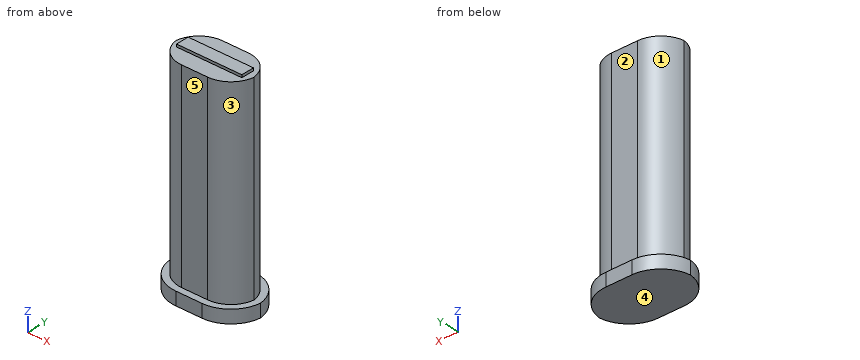
from build123d import *

# Parameters (mm, degrees)
F0_W     = 12.7
F0_H     = 2.54
F1_DEPTH = 38.608
F2_DEPTH = 38.1
F3_DEPTH = 2.54


with BuildPart() as f1:
    # F0 (on Top) → F1 (new body)
    with BuildSketch(Plane.XY):
        Rectangle(F0_W, F0_H)
    extrude(amount=F1_DEPTH)



with BuildPart() as f2:
    # F0 (on Top) → F2 (new body)
    with BuildSketch(Plane.XY):
        with BuildLine():
            Line((-2.54, -4.445), (2.54, -4.445))
            ThreePointArc((2.54, -4.445), (5.900104, -3.175), (7.580156, 0))
            ThreePointArc((7.580156, 0), (5.900104, 3.175), (2.54, 4.445))
            Line((2.54, 4.445), (-2.54, 4.445))
            ThreePointArc((-2.54, 4.445), (-5.900104, 3.175), (-7.580156, 0))
            ThreePointArc((-7.580156, 0), (-5.900104, -3.175), (-2.54, -4.445))
        make_face()
        Rectangle(F0_W, F0_H, mode=Mode.SUBTRACT)
        Rectangle(F0_W, F0_H)
    extrude(amount=F2_DEPTH)


with BuildPart() as f1_1:
    add(f1.part)

    add(f2.part)  # F3 merges F2
    # F0 (on Top) → F3 (join)
    with BuildSketch(Plane.XY):
        with BuildLine():
            Line((-2.54, -5.715), (2.54, -5.715))
            ThreePointArc((2.54, -5.715), (6.799709, -4.074286), (8.85817, 0))
            ThreePointArc((8.85817, 0), (6.799709, 4.074286), (2.54, 5.715))
            Line((2.54, 5.715), (-2.54, 5.715))
            ThreePointArc((-2.54, 5.715), (-6.799709, 4.074286), (-8.85817, 0))
            ThreePointArc((-8.85817, 0), (-6.799709, -4.074286), (-2.54, -5.715))
        make_face()
        with BuildLine():
            ThreePointArc((-7.62, 0.635), (-7.610029, 0.316876), (-7.580156, 0))
            ThreePointArc((-7.580156, 0), (-7.610029, -0.316876), (-7.62, -0.635))
            Line((-7.62, -0.635), (-7.62, 0.635))
        make_face(mode=Mode.SUBTRACT)
        with BuildLine():
            ThreePointArc((7.580156, 0), (5.900104, -3.175), (2.54, -4.445))
            Line((2.54, -4.445), (-2.54, -4.445))
            ThreePointArc((-2.54, -4.445), (-5.900104, -3.175), (-7.580156, 0))
            ThreePointArc((-7.580156, 0), (-5.900104, 3.175), (-2.54, 4.445))
            Line((-2.54, 4.445), (2.54, 4.445))
            ThreePointArc((2.54, 4.445), (5.900104, 3.175), (7.580156, 0))
        make_face(mode=Mode.SUBTRACT)
        with BuildLine():
            ThreePointArc((7.62, -0.635), (7.610029, -0.316876), (7.580156, 0))
            ThreePointArc((7.580156, 0), (7.610029, 0.316876), (7.62, 0.635))
            Line((7.62, 0.635), (7.62, -0.635))
        make_face(mode=Mode.SUBTRACT)
        with BuildLine():
            Line((-2.54, -4.445), (2.54, -4.445))
            ThreePointArc((2.54, -4.445), (5.900104, -3.175), (7.580156, 0))
            ThreePointArc((7.580156, 0), (5.900104, 3.175), (2.54, 4.445))
            Line((2.54, 4.445), (-2.54, 4.445))
            ThreePointArc((-2.54, 4.445), (-5.900104, 3.175), (-7.580156, 0))
            ThreePointArc((-7.580156, 0), (-5.900104, -3.175), (-2.54, -4.445))
        make_face()
        Rectangle(F0_W, F0_H, mode=Mode.SUBTRACT)
        Rectangle(F0_W, F0_H)
        with BuildLine():
            ThreePointArc((7.62, 0.635), (7.610029, 0.316876), (7.580156, 0))
            ThreePointArc((7.580156, 0), (7.610029, -0.316876), (7.62, -0.635))
            Line((7.62, -0.635), (7.62, 0.635))
        make_face()
        with BuildLine():
            ThreePointArc((-7.62, -0.635), (-7.610029, -0.316876), (-7.580156, 0))
            ThreePointArc((-7.580156, 0), (-7.610029, 0.316876), (-7.62, 0.635))
            Line((-7.62, 0.635), (-7.62, -0.635))
        make_face()
    extrude(amount=-F3_DEPTH)


solid = f1_1.part
The listing builds one solid part. Answer for the finished solid, in the listing's coordinates (mm). Face numbers are marked on the shaded views. A direction names the side the tool comes from. Give positions to 0.01 mm unless a question says otherwise; leave off trailing zeros. Loops run counter-clockwise (first coordinate to the right, second up) from the corner with the lowest first, then second, coordinate; pieces in that order, holes last. Notation, with made-up numbers: (-18.5, 48.5) - (-2.5, 48.5) arc R19 ccw to (-2.5, 75.5) - close; hole circle Ø11 at (-7.5, 46.25). An arc over 180 degrees is marked (long way). Answer as a JSON object with one key per item and string values.
1. A cutting plane is placed at D-D (x = -3.5). Write down the section's boundary in (y, z).
Determined:
{"outline": "(-5.64, -2.54) - (5.64, -2.54) - (5.64, 0) - (4.35, 0) - (4.35, 38.1) - (1.27, 38.1) - (1.27, 38.61) - (-1.27, 38.61) - (-1.27, 38.1) - (-4.35, 38.1) - (-4.35, 0) - (-5.64, 0) - close"}
2. For the marked faces 1, 2, 3, 4 and 5, determine the directions among +Z, -Z, +X, -X, +Y, -Y from which every point of the face is accessible in a straight line to the end or side of a thin tool.
Determined:
{"face 1": "+Z, -X, +Y", "face 2": "+Z, +X, -X, +Y", "face 3": "+Z, +X, -Y", "face 4": "-Z, +X, -X, +Y, -Y", "face 5": "+Z, +X, -X, -Y"}
3. Flat-ended cylindrical pins translate along their axes: pin 1 Ø1 at (y, z) = (4.5, 31) entering from +X; pin 2 Ø5 at (x, z) = (-1.5, 12.5) entering from -Y (3 decimals); pin 3 Ø0.6 at (x, z) = (1, 38.5) entering from -Y. Find the tip coordinate at first contact, or state that the pin passes through.
Determined:
{"pin 1": "x = 4.62", "pin 2": "y = -4.445", "pin 3": "y = -1.27"}
4. A cutting plane is placed at A-A (x = 0.5). Write down the section's boundary in (y, z) (3 decimals), then the cut area to 3 significant figures.
Determined:
{"outline": "(-5.715, -2.54) - (5.715, -2.54) - (5.715, 0) - (4.445, 0) - (4.445, 38.1) - (1.27, 38.1) - (1.27, 38.608) - (-1.27, 38.608) - (-1.27, 38.1) - (-4.445, 38.1) - (-4.445, 0) - (-5.715, 0) - close", "area": "369 mm²"}
5. A cutting plane is placed at C-C (y = -3). Write down the section's boundary in (x, z), then the cut area to 3 significant figures.
Determined:
{"outline": "(-7.75, -2.54) - (7.75, -2.54) - (7.75, 0) - (6.09, 0) - (6.09, 38.1) - (-6.09, 38.1) - (-6.09, 0) - (-7.75, 0) - close", "area": "503 mm²"}
6. A cutting plane is placed at B-B (z = 32). Write down the section's boundary in (x, y) (3 decimals).
Determined:
{"outline": "(-7.58, 0) arc R5.08 ccw to (-2.54, -4.445) - (2.54, -4.445) arc R5.08 ccw to (7.58, 0) arc R5.08 ccw to (2.54, 4.445) - (-2.54, 4.445) arc R5.08 ccw to start"}
7. Find the intervals of material crossed by L1, parallel to Z at x = -4.75, y = 1.75; L2, parallel to Z at x = 8, y = -2.25; L3, parallel to Y at x = -1.75, z = 17 (3 decimals), in increasing order. Write a range as [from, to].
Determined:
{"L1": "[-2.54, 38.1]", "L2": "[-2.54, 0]", "L3": "[-4.445, 4.445]"}
